Geometry: final body of the model. Coordinates: model frame, mm. A direction names the side the tool comes from. Give positions to 0.01 mm unless a question says otherwise; leave off trailing zeros. Loops run counter-clockwise (first coordinate to the right, second up) from the corner with the lowest first, then second, coordinate; pieces in that order, holes last.
from build123d import *

# Parameters (mm, degrees)
SKETCH_2_R               = 1.6
CUT_EXTRUDE_1_DEPTH      = 10
CUT_EXTRUDE_2_DEPTH      = 10
CUT_EXTRUDE_2_DEPTH_BACK = 10
SKETCH_3_R               = 1.55


with BuildPart() as part:
    # Sketch 1 → Revolve 1 (revolve)
    with BuildSketch(Plane.XY, mode=Mode.PRIVATE) as revolve_1_sk:
        Polygon((-2.5, 0.013967073), (-11, 0.013967073), (-11, 2.013967073), (-5, 2.013967073), (-5, 12.013967073), (-2.5, 12.013967073), align=None)
    revolve(revolve_1_sk.sketch.rotate(Axis((0, 0, 0), (0, 1, 0)), 270), axis=Axis((0, 0, 0), (0, 1, 0)))

    # Sketch 2 → Cut-Extrude 1 (cut)
    with BuildSketch(Plane.XZ.offset(-0.013967073)):
        with Locations(Location((-8, 0, 0), (0, 0, 270))):
            Circle(SKETCH_2_R)
        with Locations(Location((0, 8, 0), (0, 0, 270))):
            Circle(SKETCH_2_R)
        with Locations(Location((8, 0, 0), (0, 0, 270))):
            Circle(SKETCH_2_R)
        with Locations(Location((0, -8, 0), (0, 0, 270))):
            Circle(SKETCH_2_R)
    extrude(amount=-CUT_EXTRUDE_1_DEPTH, mode=Mode.SUBTRACT)

    # Sketch 3 → Cut-Extrude 2 (cut, two sides: drawn at the far end of the back side and taken through both)
    with BuildSketch(Plane(origin=(0, 0, 0), x_dir=(0, -1, 0), z_dir=(0.7071067811865464, 0, 0.7071067811865488)).offset(-CUT_EXTRUDE_2_DEPTH_BACK)):
        with Locations(Location((-8.513967073, 0, 0), (0, 0, 270))):
            Circle(SKETCH_3_R)
    extrude(amount=CUT_EXTRUDE_2_DEPTH + CUT_EXTRUDE_2_DEPTH_BACK, mode=Mode.SUBTRACT)


solid = part.part
Item 1: Section query A-A on z = 0. Return loops of the section in (x, y).
Values follow:
outline: (-11, 0.01) - (-9.6, 0.01) - (-9.6, 2.01) - (-11, 2.01) - close; (-6.4, 0.01) - (-2.5, 0.01) - (-2.5, 12.01) - (-5, 12.01) - (-5, 2.01) - (-6.4, 2.01) - close; (2.5, 0.01) - (6.4, 0.01) - (6.4, 2.01) - (5, 2.01) - (5, 12.01) - (2.5, 12.01) - close; (9.6, 0.01) - (11, 0.01) - (11, 2.01) - (9.6, 2.01) - close
Item 2: Section query D-D on y = 4. Return loops of the section in (x, z), plus the area to 3 significant figures.
Values follow:
outline: circle Ø10 at (0, 0); hole circle Ø5 at (0, 0)
area: 58.9 mm2
Item 3: Draft query along Z for faces 3 (the face through (4.436, 7.084, -2.307)), 4 (the face through (2.22, 5.93, -1.15)), 5 (the face through (-3, 0.014, 0)). Return one class per face: +Z half, -Z half, draft (parallel to the pull), parting line (faces both ways), or undercut.
Values follow:
face 3: parting line
face 4: undercut
face 5: draft
Item 4: Section query B-B on x = 0. Return loops of the section in (y, z), plus the area to 3 significant figures.
Values follow:
outline: (0.01, -11) - (2.01, -11) - (2.01, -9.6) - (0.01, -9.6) - close; (0.01, -6.4) - (2.01, -6.4) - (2.01, -5) - (12.01, -5) - (12.01, -2.5) - (0.01, -2.5) - close; (0.01, 2.5) - (12.01, 2.5) - (12.01, 5) - (2.01, 5) - (2.01, 6.4) - (0.01, 6.4) - close; (0.01, 9.6) - (2.01, 9.6) - (2.01, 11) - (0.01, 11) - close
area: 71.2 mm2
Item 5: Pin query (flat end, axial travel): pin 1 (1.9 mm diameter, centred on x = 8, z = 0, fed in from -Y); pin 2 (5 mm diameter, centred on x = 0, z = -8, fed in from +Y). Return the tip coordinate at first contact, or that it passes through.
Values follow:
pin 1: passes through
pin 2: stops at y = 2.01
Item 6: Section query C-C on y = 9.5. Return loops of the section in (x, z), plus the area to 3 significant figures.
Values follow:
outline: (-4.28, -2.59) - (-2.4, -0.71) arc R2.5 cw to (0.71, 2.4) - (2.59, 4.28) arc R5 ccw to start; (-2.59, -4.28) arc R5 ccw to (4.28, 2.59) - (2.4, 0.71) arc R2.5 cw to (-0.71, -2.4) - close
area: 46.7 mm2
Item 7: Ray query, probe 1 along X at (y, z) = (0.95, 0); probe 2 along Y at (x, z) = (9.5, 1.5); probe 3 along X at (y, z) = (9.5, 0). Return the intervals inside material, ascending.
Values follow:
probe 1: x = -11 to -9.6, -6.4 to -2.5, 2.5 to 6.4, 9.6 to 11
probe 2: y = 0.01 to 2.01
probe 3: x = -5 to -2.5, 2.5 to 5
Item 8: Set-up query: faces 1 (the face through (0.07, 1, 9.6)), 2 (the face through (2, 2.014, -5)). Return all of +Z, -Z, +X, -X, +Y, -Y with unobstructed straight access to the full face (end or side cutting, diameter ignored); none if empty.
Values follow:
face 1: +Y, -Y
face 2: +Y
